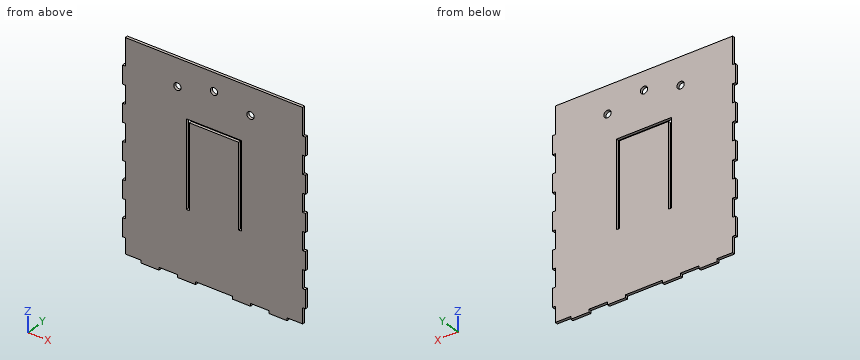
from build123d import *

# Parameters (mm, degrees)
SKETCH1_W           = 200
SKETCH1_H           = 230
BOSS_EXTRUDE1_DEPTH = 3
CUT_EXTRUDE2_DEPTH  = 3
SKETCH5_W           = 3
SKETCH5_H           = 20
SKETCH5_W_2         = 20
SKETCH5_H_2         = 3
SKETCH5_W_3         = 40
CUT_EXTRUDE4_DEPTH  = 3
SKETCH6_W           = 3
SKETCH6_H           = 5
BOSS_EXTRUDE2_DEPTH = 3
SKETCH7_W           = 3
SKETCH7_H           = 10
CUT_EXTRUDE5_DEPTH  = 3
SKETCH8_R           = 4
CUT_EXTRUDE6_DEPTH  = 3


with BuildPart() as part:
    # Sketch1 → Boss-Extrude1 (new body)
    with BuildSketch(Plane(origin=(0, 0, 0), x_dir=(1, 0, 0), z_dir=(0, 1, 0))):
        with Locations((0, -25)):
            Rectangle(SKETCH1_W, SKETCH1_H)
    extrude(amount=BOSS_EXTRUDE1_DEPTH)

    # Sketch2 → Cut-Extrude2 (cut)
    with BuildSketch(Plane(origin=(0, 3, 0), x_dir=(1, 0, 0), z_dir=(0, 1, 0))):
        Polygon((-30, -80), (30, -80), (30, 20), (27, 20), (27, -77), (-27, -77), (-27, 20), (-30, 20), align=None)
    extrude(amount=-CUT_EXTRUDE2_DEPTH, mode=Mode.SUBTRACT)

    # Sketch5 → Cut-Extrude4 (cut)
    with BuildSketch(Plane(origin=(0, 3, 0), x_dir=(1, 0, 0), z_dir=(0, 1, 0))):
        with Locations((98.5, -120)):
            Rectangle(SKETCH5_W, SKETCH5_H)
        Polygon((100, 90), (80, 90), (80, 87), (97, 87), (97, 70), (100, 70), align=None)
        Polygon((-100, 90), (-100, 70), (-97, 70), (-97, 87), (-80, 87), (-80, 90), align=None)
        with Locations((98.5, 40)):
            Rectangle(SKETCH5_W, SKETCH5_H)
        with Locations((98.5, 0)):
            Rectangle(SKETCH5_W, SKETCH5_H)
        with Locations((98.5, -40)):
            Rectangle(SKETCH5_W, SKETCH5_H)
        with Locations((98.5, -80)):
            Rectangle(SKETCH5_W, SKETCH5_H)
        with Locations((-98.5, 40)):
            Rectangle(SKETCH5_W, SKETCH5_H)
        with Locations((-98.5, 0)):
            Rectangle(SKETCH5_W, SKETCH5_H)
        with Locations((-98.5, -40)):
            Rectangle(SKETCH5_W, SKETCH5_H)
        with Locations((-98.5, -80)):
            Rectangle(SKETCH5_W, SKETCH5_H)
        with Locations((-98.5, -120)):
            Rectangle(SKETCH5_W, SKETCH5_H)
        with Locations((50, 88.5)):
            Rectangle(SKETCH5_W_2, SKETCH5_H_2)
        with Locations((0, 88.5)):
            Rectangle(SKETCH5_W_3, SKETCH5_H_2)
        with Locations((-50, 88.5)):
            Rectangle(SKETCH5_W_2, SKETCH5_H_2)
    extrude(amount=-CUT_EXTRUDE4_DEPTH, mode=Mode.SUBTRACT)

    # Sketch6 → Boss-Extrude2 (add)
    with BuildSketch(Plane(origin=(0, 3, 0), x_dir=(1, 0, 0), z_dir=(0, 1, 0))):
        with Locations((28.5, 17.5)):
            Rectangle(SKETCH6_W, SKETCH6_H)
        with Locations((-28.5, 17.5)):
            Rectangle(SKETCH6_W, SKETCH6_H)
    extrude(amount=-BOSS_EXTRUDE2_DEPTH)

    # Sketch7 → Cut-Extrude5 (cut)
    with BuildSketch(Plane(origin=(0, 3, 0), x_dir=(1, 0, 0), z_dir=(0, 1, 0))):
        with Locations((98.5, -135)):
            Rectangle(SKETCH7_W, SKETCH7_H)
        with Locations((-98.5, -135)):
            Rectangle(SKETCH7_W, SKETCH7_H)
    extrude(amount=-CUT_EXTRUDE5_DEPTH, mode=Mode.SUBTRACT)

    # Sketch8 → Cut-Extrude6 (cut)
    with BuildSketch(Plane(origin=(0, 3, 0), x_dir=(1, 0, 0), z_dir=(0, 1, 0))):
        with Locations((0, -120)):
            Circle(SKETCH8_R)
        with Locations((40, -110)):
            Circle(SKETCH8_R)
        with Locations((-40, -110)):
            Circle(SKETCH8_R)
    extrude(amount=-CUT_EXTRUDE6_DEPTH, mode=Mode.SUBTRACT)


solid = part.part
Source: CAD feature listing. Evaluate the final solid. Frame: model axes, mm. Coordinates: 2 decimals unless noted, no trailing zeros. Write each loop counter-clockwise with the first axis right and the second up, starting at its lowest first coordinate (ties: lowest second). Pieces come first, ordered by that corner, then holes. Notation, with made-up numbers: M 75,50.5 L 103,50.5 A8 ccw 103,59.5 Z; hole C -28.5,76 d3. An arc over 180 degrees is marked long. Use a Markdown table: item, result.
1) Section C-C, the plane z = 62. Output: boundary loops of the cut face in (x, y), then the cut area to 3 significant figures.
Conclusion:
| item | result |
|---|---|
| outline | M -100,0 L -30,0 L -30,3 L -100,3 Z; M -27,0 L 27,0 L 27,3 L -27,3 Z; M 30,0 L 100,0 L 100,3 L 30,3 Z |
| area | 582 mm^2 |
2) Section B-B, the plane x = 0. Output: boundary loops of the cut face in (y, z).
Conclusion:
| item | result |
|---|---|
| outline | M 0,-87 L 3,-87 L 3,77 L 0,77 Z; M 0,80 L 3,80 L 3,116 L 0,116 Z; M 0,124 L 3,124 L 3,140 L 0,140 Z |
3) Section A-A, the plane z = 120. Output: boundary loops of the cut face in (x, y), then the cut area to 3 significant figures.
Conclusion:
| item | result |
|---|---|
| outline | M -97,0 L -4,0 L -4,3 L -97,3 Z; M 4,0 L 97,0 L 97,3 L 4,3 Z |
| area | 558 mm^2 |
4) Ray query, L1, parallel to X at y = 2.7, z = 54.5; L2, parallel to Z at x = 0, y = 1.8; L3, parallel to Z at x = 14.5, y = 2.2. Return the intervals inside material, ascending.
Conclusion:
| item | result |
|---|---|
| L1 | x = -100 to -30, -27 to 27, 30 to 100 |
| L2 | z = -87 to 77, 80 to 116, 124 to 140 |
| L3 | z = -87 to 77, 80 to 140 |
5) First-contact query: pin 1 Ø1.5 at (x, y) = (-98, 1) entering from +Z; pin 2 Ø1.5 at (y, z) = (1.5, -88.5) entering from -X; pin 3 Ø1 at (y, z) = (0.5, -32.5) entering from -X. Flat tips, straight axial feed; report the tip coordinate or a pass-through.
Conclusion:
| item | result |
|---|---|
| pin 1 | stops at z = 110 |
| pin 2 | stops at x = -80 |
| pin 3 | stops at x = -97 |
6) Section D-D, the plane y = 1.55. Give the number of separate pieces and of enclosed holes in the cut face, then the cut area to 3 significant figures.
Conclusion:
| item | result |
|---|---|
| separate pieces | 1 |
| enclosed holes | 4 |
| area | 44,000 mm^2 |
